from build123d import *

# Parameters (mm, degrees)
BOX018_W               = 2.7
BOX018_H               = 2.7
BOX018_DEPTH           = 2.8
BOX021_W               = 2.7
BOX021_H               = 2.7
BOX021_DEPTH           = 2.8
BOX022_W               = 2.7
BOX022_H               = 2.7
BOX022_DEPTH           = 2.8
BOX023_W               = 2.7
BOX023_H               = 2.7
BOX023_DEPTH           = 2.8
BOX024_W               = 2.7
BOX024_H               = 2.7
BOX024_DEPTH           = 2.8
BOX025_W               = 2.7
BOX025_H               = 2.7
BOX025_DEPTH           = 2.8
BOX026_W               = 2.7
BOX026_H               = 2.7
BOX026_DEPTH           = 2.8
BOX019_W               = 2.7
BOX019_H               = 2.7
BOX019_DEPTH           = 2.8
BOX019_PLACEMENT_ANGLE = 45
BOX020_W               = 2.7
BOX020_H               = 2.7
BOX020_DEPTH           = 2.8
CYLINDER050_R          = 0.75
CYLINDER050_DEPTH      = 10
CYLINDER051_R          = 0.75
CYLINDER051_DEPTH      = 10
CYLINDER049_R          = 0.75
CYLINDER049_DEPTH      = 10
CYLINDER048_R          = 12
CYLINDER048_DEPTH      = 2.6


with BuildPart() as cube018:
    # Box018 → Box018 (new body)
    with BuildSketch(Plane(origin=(-3.6, 2.55, 2.6), x_dir=(1, 0, 0), z_dir=(0, 0, 1))):
        with Locations((1.35, 1.35)):
            Rectangle(BOX018_W, BOX018_H)
    extrude(amount=BOX018_DEPTH)


with BuildPart() as cube021:
    # Box021 → Box021 (new body)
    with BuildSketch(Plane(origin=(-6.55, -4.35, 2.6), x_dir=(1, 0, 0), z_dir=(0, 0, 1))):
        with Locations((1.35, 1.35)):
            Rectangle(BOX021_W, BOX021_H)
    extrude(amount=BOX021_DEPTH)


with BuildPart() as cube022:
    # Box022 → Box022 (new body)
    with BuildSketch(Plane(origin=(-5.85, -1.35, 2.6), x_dir=(1, 0, 0), z_dir=(0, 0, 1))):
        with Locations((1.35, 1.35)):
            Rectangle(BOX022_W, BOX022_H)
    extrude(amount=BOX022_DEPTH)


with BuildPart() as cube023:
    # Box023 → Box023 (new body)
    with BuildSketch(Plane(origin=(-6.55, 1.65, 2.6), x_dir=(1, 0, 0), z_dir=(0, 0, 1))):
        with Locations((1.35, 1.35)):
            Rectangle(BOX023_W, BOX023_H)
    extrude(amount=BOX023_DEPTH)


with BuildPart() as cube024:
    # Box024 → Box024 (new body)
    with BuildSketch(Plane(origin=(0.9, 2.55, 2.6), x_dir=(1, 0, 0), z_dir=(0, 0, 1))):
        with Locations((1.35, 1.35)):
            Rectangle(BOX024_W, BOX024_H)
    extrude(amount=BOX024_DEPTH)


with BuildPart() as cube025:
    # Box025 → Box025 (new body)
    with BuildSketch(Plane(origin=(3.85, 1.65, 2.6), x_dir=(1, 0, 0), z_dir=(0, 0, 1))):
        with Locations((1.35, 1.35)):
            Rectangle(BOX025_W, BOX025_H)
    extrude(amount=BOX025_DEPTH)


with BuildPart() as cube026:
    # Box026 → Box026 (new body)
    with BuildSketch(Plane(origin=(3.15, -1.35, 2.6), x_dir=(1, 0, 0), z_dir=(0, 0, 1))):
        with Locations((1.35, 1.35)):
            Rectangle(BOX026_W, BOX026_H)
    extrude(amount=BOX026_DEPTH)


with BuildPart() as cube019:
    # Box019 → Box019 (new body)
    with BuildSketch(Plane.XY):
        with Locations((1.35, 1.35)):
            Rectangle(BOX019_W, BOX019_H)
    extrude(amount=BOX019_DEPTH)


with BuildPart() as cube019_1:
    # Box019 placement: moved
    add(cube019.part.moved(Location((0, -7.91, 2.6))).rotate(Axis((0, -7.91, 2.6), (0, 0, 1)), BOX019_PLACEMENT_ANGLE))


with BuildPart() as fusion019:
    # Box020 → Box020 (new body)
    with BuildSketch(Plane(origin=(-3.6, -5.25, 2.6), x_dir=(1, 0, 0), z_dir=(0, 0, 1))):
        with Locations((1.35, 1.35)):
            Rectangle(BOX020_W, BOX020_H)
    extrude(amount=BOX020_DEPTH)

    # Fusion019: union Cube019
    add(cube019_1.part)


with BuildPart() as cylinder051:
    # Cylinder050 → Cylinder050 (new body)
    with BuildSketch(Plane(origin=(0, 6, 0), x_dir=(1, 0, 0), z_dir=(0, 0, 1))):
        Circle(CYLINDER050_R)
    extrude(amount=CYLINDER050_DEPTH)


with BuildPart() as cylinder048:
    # Cylinder051 → Cylinder051 (new body)
    with BuildSketch(Plane(origin=(2.25, -3.9, 0), x_dir=(1, 0, 0), z_dir=(0, 0, 1))):
        Circle(CYLINDER051_R)
    extrude(amount=CYLINDER051_DEPTH)


with BuildPart() as compound001:
    # Cylinder049 → Cylinder049 (new body)
    with BuildSketch(Plane(origin=(5.2, -3, 0), x_dir=(1, 0, 0), z_dir=(0, 0, 1))):
        Circle(CYLINDER049_R)
    extrude(amount=CYLINDER049_DEPTH)

    # Compound001: union Cube018, Cube021, Cube022, Cube023, Cube024, Cube025, Cube026, Fusion019, Cylinder051, Cylinder048
    add(cube018.part)
    add(cube021.part)
    add(cube022.part)
    add(cube023.part)
    add(cube024.part)
    add(cube025.part)
    add(cube026.part)
    add(fusion019.part)
    add(cylinder051.part)
    add(cylinder048.part)


with BuildPart() as pcb_solder_jig:
    # Cylinder048 → Cylinder048 (new body)
    with BuildSketch(Plane.XY.offset(2.7)):
        Circle(CYLINDER048_R)
    extrude(amount=CYLINDER048_DEPTH)

    # Cut013010: cut Compound001
    add(compound001.part, mode=Mode.SUBTRACT)


solid = pcb_solder_jig.part
Could you check a few things on this model? Use its own coordinates, in mm. Coordinates: 2 decimals unless noted, no trailing zeros. Order: outer loops, then holes, each group sorted by start corner. A loop starts at its lowest first (then second) coordinate and runs counter-clockwise, first axis right, second up. Notation, with made-up numbers: (3.5, -33.5) - (54.5, -33.5) arc R28 cw to (54.5, -0.5) - close; hole circle Ø6 at (56.25, 82.5). An arc over 180 degrees is marked (long way). Answer in a Markdown table with one row per item. Add a question column.
(1) Will these pins go through, and if not, where does the flat tip stop? pin 1 (1.3 mm diameter, centred on y = -3.5, z = 3.5, fed in from +X); pin 2 (0.8 mm diameter, centred on x = 2, z = 4.5, fed in from +Y); pin 3 (0.8 mm diameter, centred on x = -3, z = 4.5, fed in from -Y).
(2) If we section it at D-D, the plane z = 3.3: State how many separate pieces and enclosed holes the cut face has, then the cut area to 3 significant figures.
(3) I need wall thicknesses on L1, parallel to Y at x = 1, z = 3.7; L2, parallel to X at y = -3.5, z = 3.2; L3, parallel to X at y = -4.25, z = 4.1. Which ranges of each line are inside material? Lowest first, please.
(4) If we mould it in two halves opening along Y, with no side actions, what happens to faces 1 (the face through (-11.99, 0.53, 3.98)), 2 (the face through (6.55, 3, 4))? For each: released by +Y, released by -Y, zero draft, split by the parting line, or undercut.
(5) If we section it at B-B, the plane x = 5.2: Please give me the cut outline in (y, z).
(6) If we section it at A-A, the plane y = 0: Please give me the cut outline in (x, z).
(7) If we section it at C-C, the plane y = 6: Please give me the cut outline in (x, z).
Results are:
| question | item | result |
|---|---|---|
| 1 | pin 1 | stops at x = 11.66 |
| 1 | pin 2 | stops at y = 11.89 |
| 1 | pin 3 | stops at y = -11.71 |
| 2 | separate pieces | 1 |
| 2 | enclosed holes | 11 |
| 2 | area | 382 mm2 |
| 3 | L1 | y = -11.96 to -6.91, -5.09 to 2.55, 5.25 to 11.96 |
| 3 | L2 | x = -11.48 to -6.55, -3.85 to -3.6, -0.9 to 1.62, 2.88 to 4.64, 5.76 to 11.48 |
| 3 | L3 | x = -11.22 to -6.55, -3.85 to -3.6, -0.9 to -0.16, 0.16 to 1.59, 2.91 to 11.22 |
| 4 | face 1 | split by the parting line |
| 4 | face 2 | undercut |
| 5 | outline | (-10.81, 2.7) - (-3.75, 2.7) - (-3.75, 5.3) - (-10.81, 5.3) - close; (-2.25, 2.7) - (-1.35, 2.7) - (-1.35, 5.3) - (-2.25, 5.3) - close; (1.35, 2.7) - (1.65, 2.7) - (1.65, 5.3) - (1.35, 5.3) - close; (4.35, 2.7) - (10.81, 2.7) - (10.81, 5.3) - (4.35, 5.3) - close |
| 6 | outline | (-12, 2.7) - (-5.85, 2.7) - (-5.85, 5.3) - (-12, 5.3) - close; (-3.15, 2.7) - (3.15, 2.7) - (3.15, 5.3) - (-3.15, 5.3) - close; (5.85, 2.7) - (12, 2.7) - (12, 5.3) - (5.85, 5.3) - close |
| 7 | outline | (-10.39, 2.7) - (-0.75, 2.7) - (-0.75, 5.3) - (-10.39, 5.3) - close; (0.75, 2.7) - (10.39, 2.7) - (10.39, 5.3) - (0.75, 5.3) - close |
